For this review, use the dimensioned drawing (mm, ordinates from the lowest corner) and the shaded views. Coordinates: 2 decimals unless noted, no trailing zeros. Write each loop counter-clockwise with the first axis right and the second up, starting at its lowest first coordinate (ties: lowest second). Pieces come first, ordered by that corner, then holes. Notation, with made-up numbers: (-37, 72.25) - (-20, 72.25) arc R15 ccw to (-20, 86.25) - close; hole circle Ø8 at (57, 34). An arc over 180 degrees is marked (long way). Use one line per item in the form item = value. Start each with the question number.
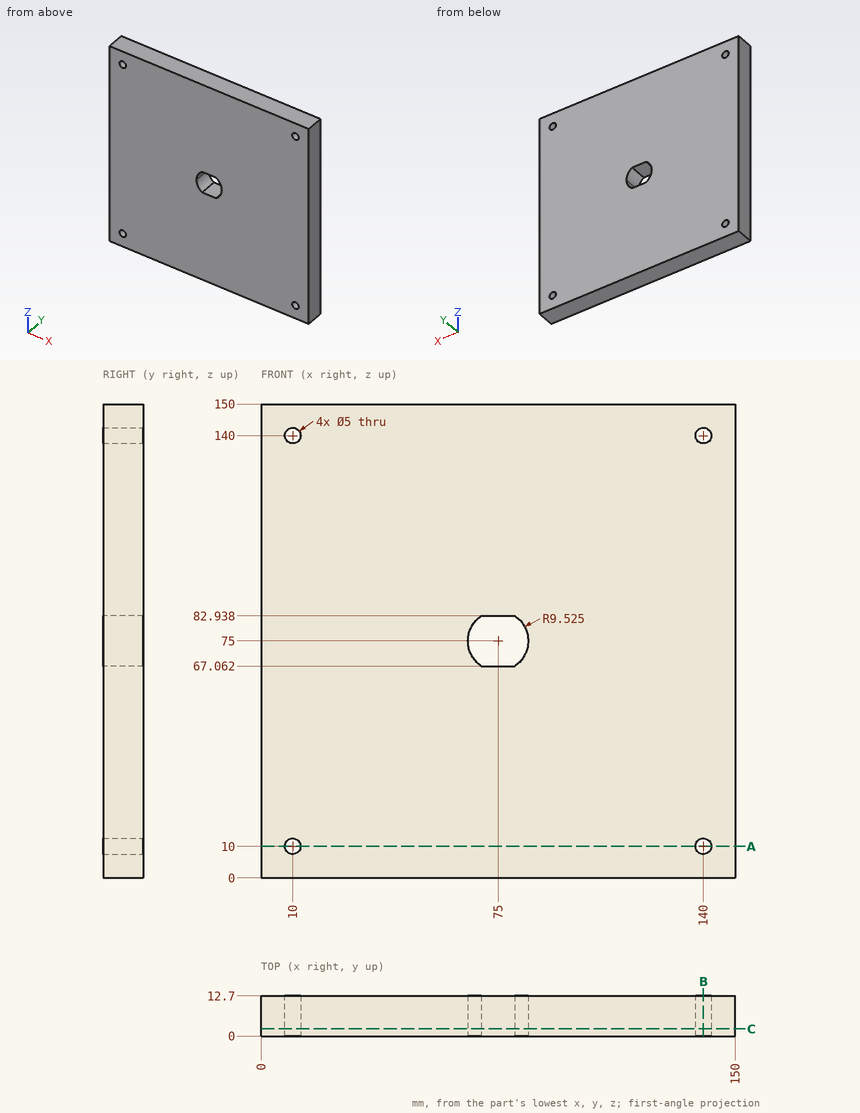
1. Take a section at C-C (y = 2.25). Count the separate pieces of the cut face and the enclosed holes in it, plus the area to 3 significant figures.
2. Take a section at B-B (x = 140). State the section outline as (y, z) points.
3. For P1, Ø4.5, axis at x = 140, z = 10, coming from the +Y side, flat-tipped, find the tip position at first contact; note if it passes through.
4. Take a section at A-A (z = 10). State the section outline as (x, y) points.
5. For L1, parallel to Z at x = 140, y = 4.5; L2, parallel to Z at x = 78.5, y = 9.5, list the stretches that pass through material, from the lowest coordinate up.
Returned:
q1.separate_pieces = 1
q1.enclosed_holes = 5
q1.area = 22,200 mm²
q2.outline = (0, 0) - (12.7, 0) - (12.7, 7.5) - (0, 7.5) - close; (0, 12.5) - (12.7, 12.5) - (12.7, 137.5) - (0, 137.5) - close; (0, 142.5) - (12.7, 142.5) - (12.7, 150) - (0, 150) - close
q3.P1 = through
q4.outline = (0, 0) - (7.5, 0) - (7.5, 12.7) - (0, 12.7) - close; (12.5, 0) - (137.5, 0) - (137.5, 12.7) - (12.5, 12.7) - close; (142.5, 0) - (150, 0) - (150, 12.7) - (142.5, 12.7) - close
q5.L1 = 0 to 7.5, 12.5 to 137.5, 142.5 to 150
q5.L2 = 0 to 67.06, 82.94 to 150
